```python
from build123d import *

# Parameters (mm, degrees)
PAD_DEPTH       = 20
SKETCH004_R     = 2
POCKET002_DEPTH = 193.001
SKETCH005_R     = 2
POCKET003_DEPTH = 85.001


with BuildPart() as part:
    # Sketch → Pad (new body)
    with BuildSketch(Plane.XY):
        Polygon((-10, -42.5), (183, -42.5), (183, -30.5), (0, -30.5), (0, 30.5), (183, 30.5), (183, 42.5), (-10, 42.5), (-10, 38.5), (-17, 38.5), (-17, 33.5), (-10, 33.5), (-10, -33.5), (-17, -33.5), (-17, -38.5), (-10, -38.5), align=None)
    extrude(amount=PAD_DEPTH)

    # Sketch004 → Pocket002 (cut, through all)
    with BuildSketch(Plane(origin=(-10, 0, 0), x_dir=(0, -1, 0), z_dir=(-1, 0, 0))):
        with Locations((0, 10)):
            Circle(SKETCH004_R)
    extrude(amount=-POCKET002_DEPTH, mode=Mode.SUBTRACT)

    # Sketch005 → Pocket003 (cut, through all)
    with BuildSketch(Plane.XZ.offset(42.5)):
        with Locations((-5, 10)):
            Circle(SKETCH005_R)
        with Locations((173, 10)):
            Circle(SKETCH005_R)
    extrude(amount=-POCKET003_DEPTH, mode=Mode.SUBTRACT)


solid = part.part
```
For this review, take the finished solid that the model builds, in its own axes (mm). A direction names the side the tool comes from. Round coordinates to 2 decimals unless told otherwise and drop trailing zeros. Loops run counter-clockwise (first coordinate to the right, second up) from the corner with the lowest first, then second, coordinate; pieces in that order, holes last.
Q1. Add section A-A on x = 173. Write out the cut boundary in (y, z), plus the area to 3 significant figures.
Result sheet:
outline: (-42.5, 0) - (-30.5, 0) - (-30.5, 8) - (-42.5, 8) - close; (-42.5, 12) - (-30.5, 12) - (-30.5, 20) - (-42.5, 20) - close; (30.5, 0) - (42.5, 0) - (42.5, 8) - (30.5, 8) - close; (30.5, 12) - (42.5, 12) - (42.5, 20) - (30.5, 20) - close
area: 384 mm2
Q2. Machinability: for faces 3 (the face through (-14, -38.5, 10)), 4 (the face through (90, 30.5, 10)), 5 (the face through (-14, 33.5, 10)), which of the approach directions +Z, -Z, +X, -X, +Y, -Y give a long, thin tool a straight path to every point of the face, cutting with its end or side? Answer none if there is none.
Result sheet:
face 3: +Z, -Z, -X, -Y
face 4: +Z, -Z, +X
face 5: +Z, -Z, -X
Q3. To check wall thickness, follow line 1 along Z through (x, y) = (173, 33); line 2 along Y through (x, z) = (21, 18.25); line 3 along X through (y, z) = (36.5, 11.5). State the ranges of each line that lie inside material, in increasing order.
Result sheet:
line 1: z = 0 to 8, 12 to 20
line 2: y = -42.5 to -30.5, 30.5 to 42.5
line 3: x = -17 to -6.32, -3.68 to 171.68, 174.32 to 183
Q4. Mouldability with a two-part tool opening along Z and no side actions: class faces 1 (the face through (-5, -22, 12)), 2 (the face through (-10, 0.5, 12.1)) as +Z half, -Z half, draft (parallel to the pull), parting line (faces both ways), or undercut.
Result sheet:
face 1: undercut
face 2: draft
Q5. Add section B-B on y = -11.5. Write out the cut boundary in (x, z).
Result sheet:
outline: (-10, 0) - (0, 0) - (0, 20) - (-10, 20) - close; hole circle Ø4 at (-5, 10)
Q6. Insertion check: pin 1 Ø3.5 at (x, z) = (-14.5, 8.5) entering from -Y; pin 2 Ø1.2 at (y, z) = (40, 9) entering from -X; pin 3 Ø2 at (x, z) = (-14, 11) entering from +Y. Each pin has a flat end and moves straight along its axis. Give the tip position at first contact, or say it passes through.
Result sheet:
pin 1: stops at y = -38.5
pin 2: stops at x = -10
pin 3: stops at y = 38.5
Q7. Add section D-D on z = 17.5. Write out the cut boundary in (x, y), plus the area to 3 significant figures.
Result sheet:
outline: (-17, -38.5) - (-10, -38.5) - (-10, -42.5) - (183, -42.5) - (183, -30.5) - (0, -30.5) - (0, 30.5) - (183, 30.5) - (183, 42.5) - (-10, 42.5) - (-10, 38.5) - (-17, 38.5) - (-17, 33.5) - (-10, 33.5) - (-10, -33.5) - (-17, -33.5) - close
area: 5,310 mm2
Q8. Add section C-C on x = 71. Write out the cut boundary in (y, z), plus the area to 3 significant figures.
Result sheet:
outline: (-42.5, 0) - (-30.5, 0) - (-30.5, 20) - (-42.5, 20) - close; (30.5, 0) - (42.5, 0) - (42.5, 20) - (30.5, 20) - close
area: 480 mm2
